Autodesk Inventor part; units mm, degrees
ref_plane "YZ Plane" through (0, 0, 0) normal (1, 0, 0) x (0, 1, 0)
ref_plane "XZ Plane" through (0, 0, 0) normal (0, 1, 0) x (-1, 0, 0)
ref_plane "XY Plane" through (0, 0, 0) normal (0, 0, 1) x (1, 0, 0)
sketch "Sketch1" plane through (0, 0, 0) normal (1, 0, 0) x (0, 1, 0)
  circle A0 centre (0, 0) radius 16.575
  line L0 (0, 16.575) -> (0, -49.725)
  line L1 (0, -33.15) -> (0, -15.05)
  line L2 (0, -15.05) -> (0, -70.05)
  line L3 (10, -70.05) -> (-10, -70.05)
  line L4 (-10, -70.05) -> (-10, -15.05)
  line L5 (-10, -15.05) -> (10, -15.05)
  line L6 (10, -15.05) -> (10, -70.05)
  line L7 (10, -70.05) -> (-10, -15.05) construction
  line L8 (-10, -70.05) -> (10, -15.05) construction
  line L9 (10, -62.65) -> (-10, -62.65)
  line L10 (-10, -62.65) -> (-10, -22.45)
  line L11 (-10, -22.45) -> (10, -22.45)
  line L12 (10, -22.45) -> (10, -62.65)
  line L13 (10, -62.65) -> (-10, -22.45) construction
  line L14 (-10, -62.65) -> (10, -22.45) construction
  line L15 (-4.95, -27.2) -> (-4.95, -17.7)
  line L16 (-4.95, -17.7) -> (4.95, -17.7)
  line L17 (4.95, -27.2) -> (-4.95, -17.7) construction
  line L18 (-4.95, -27.2) -> (4.95, -17.7) construction
  line L19 (4.95, -67.4) -> (-4.95, -67.4)
  line L20 (-4.95, -67.4) -> (-4.95, -57.9)
  line L21 (-4.95, -57.9) -> (4.95, -57.9)
  line L22 (4.95, -67.4) -> (-4.95, -57.9) construction
  line L23 (-4.95, -67.4) -> (4.95, -57.9) construction
  circle A1 centre (4.95, -17.7) radius 1.5
  circle A2 centre (-4.95, -17.7) radius 1.5
  circle A3 centre (4.95, -67.4) radius 1.5
  circle A4 centre (-4.95, -67.4) radius 1.5
  circle A5 centre (0, -33.15) radius 6.8
  line L24 (0, -80) -> (0, -55)
  arc A6 (-25, -55) -> (25, -55) centre (0, -55) ccw
  line L25 (0, 0) -> (0, 45)
  line L26 (25, 45) -> (-25, 45)
  line L27 (25, 45) -> (25, -55)
  line L28 (-25, 45) -> (-25, -55)
  circle A7 centre (0, 0) radius 7.5
  point P0 (0, -42.55)
  point P1 (0, -42.55)
  point P2 (0, -22.45)
  point P3 (0, -62.65)
  dimension "d0" = 33.15
  dimension "d2" = 66.3
  dimension "d4" = 18.1
  dimension "d5" = 55
  dimension "d6" = 20
  dimension "d7" = 55
  dimension "d8" = 40.2
  dimension "d9" = 9.9
  dimension "d10" = 9.5
  dimension "d11" = 9.9
  dimension "d12" = 9.5
  dimension "d13" = 3
  dimension "d14" = 3
  dimension "d15" = 3
  dimension "d16" = 3
  dimension "d17" = 13.6
  dimension "d20" = 25
  dimension "d21" = 45
  dimension "d22" = 15
extrude "Extrusion1" add sketch "Sketch1" along normal blind 5 contours A0 L5 L0 A7 | A0 L25 L26 L27 A6 L24 L3 L6 L5 | L0 A7 L5 A0 | A0 L5 L4 L3 L24 A6 L28 L26 L25 | L5 L6 L11 L0 A0 | A0 L0 L5 | L5 L0 A0 | A0 L0 L16 A2 L15 L11 L4 L5 | L0 L11 L15 A2 L16 | L6 L9 L2 L0 A5 L11 | L11 L0 A5 L2 L21 L20 L9 L4 | L6 L3 L2 L9 | L9 L20 A4 L19 L2 L3 L4 | L9 L20 L21 L2 | L2 L19 A4 L20 L9
sketch "Sketch2" plane through (0, 0, 0) normal (-1, 0, 0) x (0, 0, 1)
  line L0 (45, 25) -> (45, -25)
  line L1 (-55, 25) -> (45, 25)
  line L2 (45, 25) -> (-5, 25)
  line L3 (45, 25) -> (45, -25)
  arc A0 (45, -25) -> (-5, 25) centre (-5, -25) ccw
extrude "Extrusion2" cut sketch "Sketch2" against normal blind 5
sketch "Sketch3" plane through (0, 0, 0) normal (-1, 0, 0) x (0, 0, 1)
  arc A0 (45, -25) -> (-5, 25) centre (-5, -25) ccw
  arc A1 (-55, 25) -> (-55, -25) centre (-55, 0) ccw
  line L0 (45, -25) -> (-55, -25)
  line L1 (45, -25) -> (45, -50)
  line L2 (45, -50) -> (17, -50)
  line L3 (17, -50) -> (-62.8113, -23.7483)
  line L4 (45, -25) -> (-55, -25)
  arc A2 (-62.8113, -23.7483) -> (-55, -25) centre (-55, 0) ccw
  dimension "d27" = 25
  dimension "d28" = 28
extrude "Extrusion3" add sketch "Sketch3" against normal blind 5
sketch "Sketch4" plane through (0, 0, 0) normal (-1, 0, 0) x (0, 0, 1)
  circle A0 centre (0, 0) radius 7.5
  arc A1 (45, -25) -> (-5, 25) centre (-5, -25) ccw
  line L0 (-55, 25) -> (-5, 25)
  arc A2 (-55, 25) -> (-62.8113, -23.7483) centre (-55, 0) ccw
  line L1 (-62.8113, -23.7483) -> (17, -50)
  line L2 (17, -50) -> (45, -50)
  line L3 (45, -50) -> (45, -25)
  circle A3 centre (-33.15, 0) radius 6.8
  circle A4 centre (-67.4, -4.95) radius 1.5
  circle A5 centre (-67.4, 4.95) radius 1.5
  circle A6 centre (-17.7, -4.95) radius 1.5
  circle A7 centre (-17.7, 4.95) radius 1.5
extrude "Extrusion4" add sketch "Sketch4" along normal blind 3
sketch "Sketch5" plane through (-3, 0, 0) normal (-1, 0, 0) x (0, 0, 1)
  circle A0 centre (-33.15, 0) radius 6.8
  circle A1 centre (-17.7, -4.95) radius 1.5
  circle A2 centre (-67.4, 4.95) radius 1.5
  line L0 (-67.4, 4.95) -> (-17.7, 4.95)
  line L1 (-17.7, 4.95) -> (-17.7, -4.95)
  line L2 (-17.7, -4.95) -> (-67.4, -4.95)
  line L3 (-67.4, -4.95) -> (-67.4, 4.95)
  line L4 (-67.4, 0) -> (-17.7, 0)
  line L5 (-22.3, 10) -> (-62.8, 10)
  line L6 (-62.8, 10) -> (-62.8, -10)
  line L7 (-62.8, -10) -> (-22.3, -10)
  line L8 (-22.3, -10) -> (-22.3, 10)
  line L9 (-22.3, 10) -> (-62.8, -10) construction
  line L10 (-62.8, 10) -> (-22.3, -10) construction
  point P0 (-42.55, 0)
  dimension "d33" = 40.5
  dimension "d34" = 20
extrude "Extrusion5" cut sketch "Sketch5" against normal blind 3 contours L4 L8 L2 A0 | A0 L0 L8 L4 | A0 L0 L6 L5 L8 | L2 L8 L7 L6 A0 | L4 L6 L0 A0 | A0 L2 L6 L4
sketch "Sketch6" plane through (0, 0, 0) normal (-1, 0, 0) x (0, 0, 1)
  circle A0 centre (-33.15, 0) radius 6.8
  line L0 (-62.8, 10) -> (-22.3, 10)
  line L1 (-62.8, -10) -> (-62.8, 10)
  line L2 (-22.3, -10) -> (-62.8, -10)
  line L3 (-22.3, 10) -> (-22.3, -10)
  point P0 (0, 0)
extrude "Extrusion6" cut sketch "Sketch6" against normal blind 1
sketch "Sketch7" plane through (-3, 0, 0) normal (-1, 0, 0) x (0, 0, 1)
  circle A0 centre (0, 0) radius 7.5
  circle A1 centre (0, 0) radius 5
  dimension "d39" = 10
extrude "Extrusion7" add sketch "Sketch7" against normal blind 3
fillet "Fillet1" radius 1 4 edges at (-1, -10, -22.3) (-1, 10, -22.3) (-1, 10, -62.8) (-1, -10, -62.8)
properties part number "packa_strana(a)"
Build history of the part. All positions in model axes, mm. A direction names the side the tool comes from. Give positions to 0.01 mm unless a question says otherwise; leave off trailing zeros. Order: outer loops, then holes, each group sorted by start corner. A loop starts at its lowest first (then second) coordinate and runs counter-clockwise, first axis right, second up. Notation, with made-up numbers: M 84.25,0 L 91.25,0 A12 ccw 91.25,13 Z; hole C 89.25,8.25 d3. An arc over 180 degrees is marked long. Use one line per item in the form item = value.
Q1. Slice it at A-A, the plane y = 0. Write the cut outline in (x, z), and give its area (3 significant figures).
Conclusion:
outline = M -3,-80 L 5,-80 L 5,-39.95 L 1,-39.95 L 1,-62.8 L -3,-62.8 Z; M -3,-22.3 L 1,-22.3 L 1,-26.35 L 5,-26.35 L 5,-7.5 L 0,-7.5 L 0,-5 L -3,-5 Z; M -3,5 L 0,5 L 0,7.5 L 5,7.5 L 5,38.3 L -3,38.3 Z
area = 625 mm2
Q2. Pull direction Z, two halves, no side cores. Call faces 4 (the cylindrical face through (-1.48, 3.47, -79.76)), 5 (the flat face through (5, -12, -18)), 6 (the flat face through (-1, 0, -22.3)), 7 (the cylindrical face through (1.06, -3.56, -66.84)): released by +Z, released by -Z, zero draft, split by the parting line, or undercut.
Conclusion:
face_4 = released by -Z
face_5 = zero draft
face_6 = undercut
face_7 = undercut
Q3. Which spindle directions (+Z, -Z, +X, -X, +Y, -Y) get a long thin tool onto all of the face, cutting with end or side? Do faces 1 (the cylindrical face through (2.54, -1.63, -7.32)), 2 (the flat face through (-1, -10, -43)), 3 (the cylindrical face through (-1.52, -4.88, -1.08)). Say none if no direction does.
Conclusion:
face_1 = +X
face_2 = -X
face_3 = +X, -X
Q4. Slice it at C-C, the plane x = 3.75. Write the cut outline in (y, z).
Conclusion:
outline = M -50,17 L -23.75,-62.81 A25 ccw 25,-55 L 25,-5 A50 ccw -25,45 L -50,45 Z; hole C 0,0 d15; hole C 0,-33.15 d13.6; hole C -4.95,-67.4 d3; hole C -4.95,-17.7 d3; hole C 4.95,-67.4 d3; hole C 4.95,-17.7 d3
Q5. Wall check: probe 1 along Z at (x, y) = (2.25, 4.95); probe 2 along Z at (x, y) = (4.5, 6); probe 3 along Y at (x, z) = (2.75, -17.7). Give the ranges that are in metal, low to high.
Conclusion:
probe_1 = -79.51 to -68.9, -65.9 to -37.81, -28.49 to -19.2, -16.2 to -5.63, 5.63 to 35.04
probe_2 = -79.27 to -68.47, -66.33 to -36.35, -29.95 to -18.77, -16.63 to -4.5, 4.5 to 34.23
probe_3 = -38.59 to -6.45, -3.45 to 3.45, 6.45 to 25
Q6. Slice it at B-B, the plane z = -28.5. Write the cut outline in (x, y).
Conclusion:
outline = M -3,-35.03 L 5,-35.03 L 5,-4.96 L 1,-4.96 L 1,-10 L -3,-10 Z; M -3,10 L 1,10 L 1,4.96 L 5,4.96 L 5,25 L -3,25 Z
Q7. Slice it at D-D, the plane z = -70.5. Write the cut outline in (x, y).
Conclusion:
outline = M -3,-19.62 L 5,-19.62 L 5,19.62 L -3,19.62 Z
Q8. Pin check, flat tips, straight feed: P1, Ø13.5, axis at y = 0, z = 0, coming from the +X side; P2, Ø3, axis at x = 2.5, y = -12, coming from the -Z side; P3, Ø1.2, axis at x = -0.5, z = -47, coming from the -Y side. Stop position of each tip, or through.
Conclusion:
P1 = 0
P2 = -77.69
P3 = -29.15
